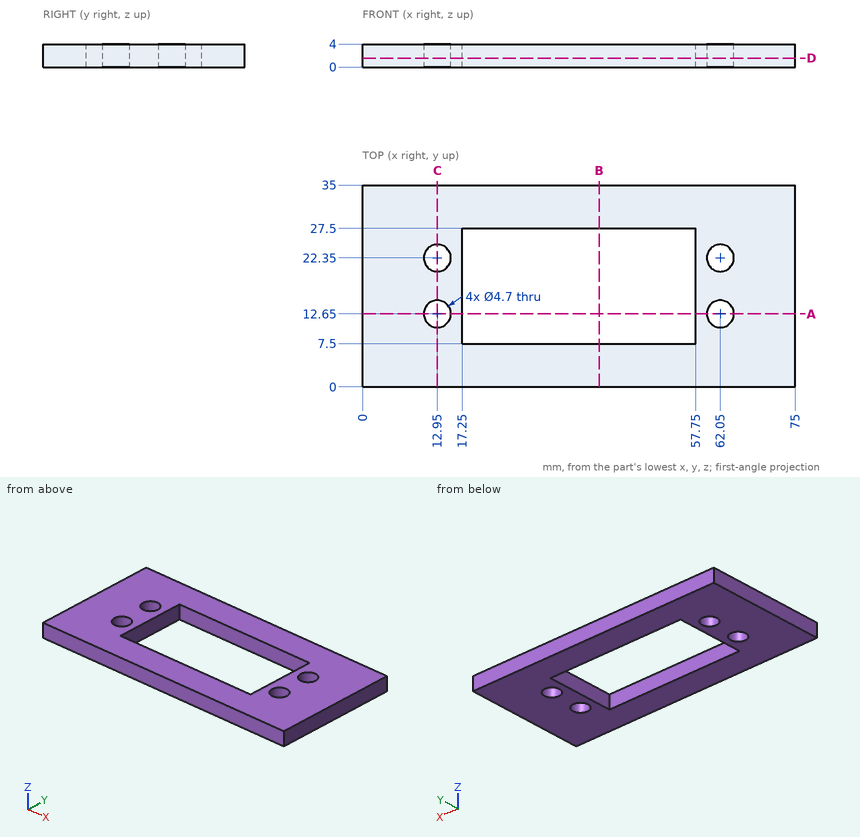
Print and shaded views of the part. All mm, measured from the part's lowest x, y and z. Round coordinates to 2 decimals unless told otherwise and drop trailing zeros. Write each loop counter-clockwise with the first axis right and the second up, starting at its lowest first coordinate (ties: lowest second). Pieces come first, ordered by that corner, then holes.
Item 1: Drop a flat-ended pin along its axis: pin 1 Ø1.5 at (x, z) = (54.5, 3) entering from -Y. Give the stop position or say it passes through.
Results:
pin 1: stops at y = 0
Item 2: Cut at A-A, the plane y = 12.65. Give the cut face in (x, z).
Results:
outline: (0, 0) - (10.6, 0) - (10.6, 4) - (0, 4) - close; (15.3, 0) - (17.25, 0) - (17.25, 4) - (15.3, 4) - close; (57.75, 0) - (59.7, 0) - (59.7, 4) - (57.75, 4) - close; (64.4, 0) - (75, 0) - (75, 4) - (64.4, 4) - close
Item 3: Cut at D-D, the plane z = 1.55. Give the cut face in (x, y), plus the area to 3 significant figures.
Results:
outline: (0, 0) - (75, 0) - (75, 35) - (0, 35) - close; hole circle Ø4.7 at (12.95, 12.65); hole circle Ø4.7 at (12.95, 22.35); hole (17.25, 7.5) - (57.75, 7.5) - (57.75, 27.5) - (17.25, 27.5) - close; hole circle Ø4.7 at (62.05, 12.65); hole circle Ø4.7 at (62.05, 22.35)
area: 1,750 mm2
Item 4: Cut at B-B, the plane x = 41. Give the cut face in (y, z).
Results:
outline: (0, 0) - (7.5, 0) - (7.5, 4) - (0, 4) - close; (27.5, 0) - (35, 0) - (35, 4) - (27.5, 4) - close
Item 5: Cut at C-C, the plane x = 12.95. Give the cut face in (y, z), plus the area to 3 significant figures.
Results:
outline: (0, 0) - (10.3, 0) - (10.3, 4) - (0, 4) - close; (15, 0) - (20, 0) - (20, 4) - (15, 4) - close; (24.7, 0) - (35, 0) - (35, 4) - (24.7, 4) - close
area: 102 mm2
Item 6: Probe L1, parallel to Y at x = 12.95, z = 2; L2, parallel to Y at x = 44.5, z = 1.55; L3, parallel to X at y = 18.5, z = 1.1. List the from-to ranges inside material, lowest first.
Results:
L1: y = 0 to 10.3, 15 to 20, 24.7 to 35
L2: y = 0 to 7.5, 27.5 to 35
L3: x = 0 to 17.25, 57.75 to 75
